Model file for the job. Use its own axes, mm. Face numbers are marked on the shaded views. A direction names the side the tool comes from. Give positions to 0.01 mm unless a question says otherwise; leave off trailing zeros. Order: outer loops, then holes, each group sorted by start corner. A loop starts at its lowest first (then second) coordinate and runs counter-clockwise, first axis right, second up. Notation, with made-up numbers: (-27.5, 70.5) -> (-11.5, 70.5) arc R28 cw to (-11.5, 93.5) -> close; hole circle Ø8 at (54.5, 56). An arc over 180 degrees is marked (long way). Answer in a Markdown table with one row per item. Add a question column.
from build123d import *

# Parameters (mm, degrees)
BOSS_EXTRUDE1_DEPTH      = 1
FILLET1_R                = 0.3
BOSS_EXTRUDE2_DEPTH      = 10
BOSS_EXTRUDE2_DEPTH_BACK = 2.3
SKETCH6_R                = 0.23
SKETCH_2_R               = 3.1
EXTRUDE_1_DEPTH          = 1.2
SKETCH_3_W               = 2.8
SKETCH_3_H               = 2.8
EXTRUDE_2_DEPTH          = 1


with BuildPart() as part:
    # Sketch1 → Boss-Extrude1 (new body)
    with BuildSketch(Plane(origin=(0, 0, 0), x_dir=(1, 0, 0), z_dir=(0, 1, 0))):
        with BuildLine():
            Line((2.942495814, -3.499271693), (3.55315323, -4.10992911))
            Line((3.55315323, -4.10992911), (4.10992911, -3.55315323))
            Line((4.10992911, -3.55315323), (3.499271693, -2.942495814))
            ThreePointArc((3.499271693, -2.942495814), (-3.232892204, 3.232892204), (2.942495814, -3.499271693))
        make_face()
    extrude(amount=-BOSS_EXTRUDE1_DEPTH)

    # Sketch5 → Revolve4 (revolve)
    with BuildSketch(Plane.XY):
        Polygon((4.1275, 4.3), (2.9718, 4.3), (2.9718, 3.8936), (3.7211, 3.8936), (3.7211, 0.8936), (0, 0.8936), (0, 0), (4.1275, 0), align=None)
    revolve(axis=Axis((0, 0.8936, 0), (0, -1, 0)))

    # Fillet1
    fillet1_edges = [part.edges().sort_by_distance(p)[0] for p in [
        (-4.1275, 0, 0),
        (-4.1275, 4.3, 0),
    ]]
    fillet(fillet1_edges, radius=FILLET1_R)

    # Sketch6 → Boss-Extrude2 (add, two sides: drawn at the far end of the back side and taken through both)
    with BuildSketch(Plane.XZ.offset(1).offset(-BOSS_EXTRUDE2_DEPTH_BACK)):
        with Locations(Location((0, -2.54, 0), (0, 0, 270))):
            Circle(SKETCH6_R)
        with Locations(Location((-2.54, 0, 0), (0, 0, 270))):
            Circle(SKETCH6_R)
        with Locations(Location((0, 2.54, 0), (0, 0, 270))):
            Circle(SKETCH6_R)
        with Locations(Location((2.54, 0, 0), (0, 0, 270))):
            Circle(SKETCH6_R)
    extrude(amount=BOSS_EXTRUDE2_DEPTH + BOSS_EXTRUDE2_DEPTH_BACK)

    # Эскиз2 → Бобышка-Вытянуть1 (add)
    with BuildSketch(Plane(origin=(0, 1.3, 0), x_dir=(1, 0, 0), z_dir=(0, 1, 0))):
        with Locations(Location((0, 0, 0), (0, 0, 270))):
            Circle(SKETCH_2_R)
    extrude(amount=EXTRUDE_1_DEPTH)

    # Эскиз3 → Бобышка-Вытянуть2 (add)
    with BuildSketch(Plane(origin=(0, 2.5, 0), x_dir=(1, 0, 0), z_dir=(0, 1, 0))):
        Rectangle(SKETCH_3_W, SKETCH_3_H)
    extrude(amount=EXTRUDE_2_DEPTH)


solid = part.part
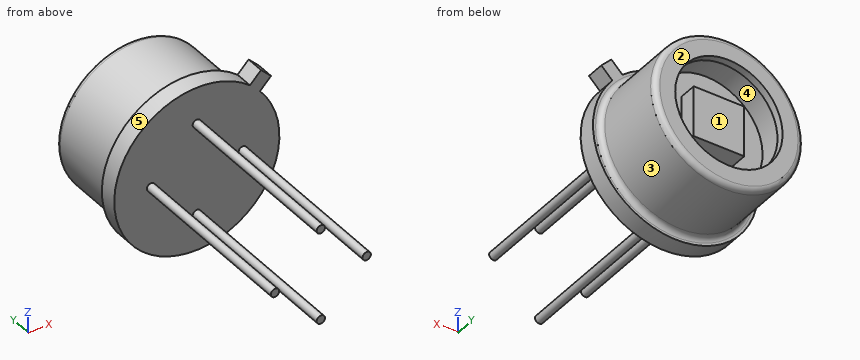
Item 1: Saw through at A-A on y = -2. List the corners of the cut face in (x, z), plus the area to 3 significant figures.
Item 2: Wall check: line 1 (Y direction, x = 2.75, z = -1.5); line 2 (Y direction, x = 0.5, z = 0); line 3 (Z direction, x = 0, y = 2.6). Give the ranges that are in metal, low to high.
Item 3: Which spindle directions (+Z, -Z, +X, -X, +Y, -Y) get a long thin tool onto all of the face, cutting with end or side? Do the marked faces 4 and 5. Say none if no direction does.
Item 4: Pin check, flat tips, straight feed: pin 1 Ø4.5 at (x, z) = (-1, -2) entering from -Y; pin 2 Ø1 at (x, z) = (-1.5, -1) entering from -Y; pin 3 Ø1.9 at (x, z) = (-0.5, -0.5) entering from +Y; pin 4 Ø0.5 at (x, y) = (0, 3) entering from -Z. Stop position of each tip, or through.
Item 5: Two-plate mould, pull along X, no slides. Class the marked faces 1, 2 and 3: pulls with the +X half, pulls with the -X half, needs draft (parallel to the pull), parting line crosses it, or undercut.
Evaluation:
| question | item | result |
|---|---|---|
| 1 | outline | circle Ø0.46 at (-2.54, 0); circle Ø0.46 at (0, -2.54); circle Ø0.46 at (0, 2.54); circle Ø0.46 at (2.54, 0) |
| 1 | area | 0.665 mm2 |
| 2 | line 1 | y = -1 to 0.89, 3.89 to 4.3 |
| 2 | line 2 | y = -1 to 0.89, 1.3 to 3.5 |
| 2 | line 3 | z = -4.13 to -3.72, -1.4 to 1.4, 3.72 to 4.13 |
| 3 | face 4 | none |
| 3 | face 5 | +Y, -Y |
| 4 | pin 1 | stops at y = -11 |
| 4 | pin 2 | stops at y = -1 |
| 4 | pin 3 | stops at y = 3.5 |
| 4 | pin 4 | stops at z = -4.13 |
| 5 | face 1 | undercut |
| 5 | face 2 | needs draft |
| 5 | face 3 | parting line crosses it |
